Here's how the part is built. I have some questions about the finished solid (model axes, mm). A direction names the side the tool comes from. Give positions to 0.01 mm unless a question says otherwise; leave off trailing zeros. Write each loop counter-clockwise with the first axis right and the second up, starting at its lowest first coordinate (ties: lowest second). Pieces come first, ordered by that corner, then holes. Notation, with made-up numbers: (-24, -38.5) -> (9, -38.5) arc R27 cw to (9, -8.5) -> close; hole circle Ø8 at (73.25, 34.5). An arc over 180 degrees is marked (long way). Return JSON: item names as keys, results as strings.
from build123d import *

# Parameters (mm, degrees)
F1_DEPTH = 914.4
F2_R     = 2.6162
F3_DEPTH = 3.176


with BuildPart() as f1:
    # F0 (on Front) → F1 (new body)
    with BuildSketch(Plane.XZ):
        with BuildLine():
            Line((-25.4, 0), (0, 0))
            ThreePointArc((0, 0), (-0.929936, 2.245064), (-3.175, 3.175))
            Line((-3.175, 3.175), (-19.05, 3.175))
            ThreePointArc((-19.05, 3.175), (-21.295064, 4.104936), (-22.225, 6.35))
            Line((-22.225, 6.35), (-22.225, 22.225))
            ThreePointArc((-22.225, 22.225), (-23.154936, 24.470064), (-25.4, 25.4))
            Line((-25.4, 25.4), (-25.4, 0))
        make_face()
    extrude(amount=F1_DEPTH)

    # F2 (on face) → F3 (cut, through all)
    with BuildSketch(Plane.XY.offset(3.175)):
        with Locations((-11.1125, -900.1125)):
            Circle(F2_R)
        with Locations((-11.1125, -14.2875)):
            Circle(F2_R)
    extrude(amount=-F3_DEPTH, mode=Mode.SUBTRACT)


solid = f1.part
1. Suppose I cut it at A-A, the plane y = -736. List the corners of the cut face in (x, z) for me (3 decimals).
Taken from the geometry:
{"outline": "(-25.4, 0) -> (0, 0) arc R3.175 ccw to (-3.175, 3.175) -> (-19.05, 3.175) arc R3.175 cw to (-22.225, 6.35) -> (-22.225, 22.225) arc R3.175 ccw to (-25.4, 25.4) -> close"}
2. Suppose I cut it at B-B, the plane z = 12. List the corners of the cut face in (x, y) for me (3 decimals), and give its area (3 significant figures).
Taken from the geometry:
{"outline": "(-25.4, -914.4) -> (-22.225, -914.4) -> (-22.225, 0) -> (-25.4, 0) -> close", "area": "2,900 mm²"}
3. If I drill on line 1 (Z direction, x = -2.75, y = -64); line 2 (Z direction, x = -17.5, y = -846.5) (3 decimals); line 3 (X direction, y = -538, z = 12) (3 decimals), over which ranges is the centre line in solid material (lowest first)? Write a range as [from, to].
Taken from the geometry:
{"line 1": "z = [0, 3.15]", "line 2": "z = [0, 3.175]", "line 3": "x = [-25.4, -22.225]"}
4. For pin 1 Ø5 at (x, y) = (-13, -291) entering from +Z (3 decimals); pin 2 Ø12 at (x, y) = (-18.5, -225.5) entering from +Z; pin 3 Ø12.5 at (y, z) = (-316.5, 12.5) entering from +X, each with a flat end and sliding along its axis, tell me the tip position at first contact or that it passes through.
Taken from the geometry:
{"pin 1": "stops at z = 3.175", "pin 2": "stops at z = 25.27", "pin 3": "stops at x = -22.22"}
5. Which directions (+Z, -Z, +X, -X, +Y, -Y) give clear straight access to the entire face, cutting with the end or side of a thin tool? Please do faces 1 (the face through (-11, -451, 3.175)), 2 (the face through (-13, -451, 0)).
Taken from the geometry:
{"face 1": "+Z, +X, +Y, -Y", "face 2": "-Z, +X, -X, +Y, -Y"}
